from build123d import *

# Parameters (mm, degrees)
F0_R     = 1.5
F0_W     = 15
F0_H     = 49.5
F1_DEPTH = 4.5
F2_R     = 2
F3_R     = 1.5
F4_DEPTH = 2
F5_W     = 4
F5_H     = 29.5
F6_DEPTH = 6.501
F7_R     = 1.5
F8_R     = 6
F9_DEPTH = 0.5


with BuildPart() as f1:
    # F0 (on Front) → F1 (new body)
    with BuildSketch(Plane.XZ):
        with BuildLine():
            ThreePointArc((-76.25, -24.75), (-72.25, -28.75), (-68.25, -24.75))
            Line((-68.25, -24.75), (-68.25, 24.75))
            Line((-68.25, 24.75), (-68.25, 26.75))
            Line((-68.25, 26.75), (40.25, 26.75))
            Line((40.25, 26.75), (40.25, 24.75))
            Line((40.25, 24.75), (40.25, -24.75))
            ThreePointArc((40.25, -24.75), (41.4215728753, -27.5784271247), (44.25, -28.75))
            Line((44.25, -28.75), (72.25, -28.75))
            ThreePointArc((72.25, -28.75), (75.0784271247, -27.5784271247), (76.25, -24.75))
            Line((76.25, -24.75), (76.25, 27))
            ThreePointArc((76.25, 27), (75.0784271247, 29.8284271247), (72.25, 31))
            Line((72.25, 31), (-72.25, 31))
            ThreePointArc((-72.25, 31), (-75.0784271247, 29.8284271247), (-76.25, 27))
            Line((-76.25, 27), (-76.25, -24.75))
        make_face()
        with Locations((-72.25, -24.75)):
            Circle(F0_R, mode=Mode.SUBTRACT)
        with Locations((72.25, -24.75)):
            Circle(F0_R, mode=Mode.SUBTRACT)
        with Locations((60.75, 0)):
            Rectangle(F0_W, F0_H, mode=Mode.SUBTRACT)
        with Locations((-72.25, 24.75)):
            Circle(F0_R, mode=Mode.SUBTRACT)
        with Locations((72.25, 24.75)):
            Circle(F0_R, mode=Mode.SUBTRACT)
    extrude(amount=F1_DEPTH)

    # F2
    f2_edges = [f1.edges().sort_by_distance(p)[0] for p in [
        (-68.25, -2.25, -24.75),
        (40.25, -2.25, -24.75),
        (68.25, -2.25, 24.75),
        (53.25, -2.25, 24.75),
        (53.25, -2.25, -24.75),
        (68.25, -2.25, -24.75),
    ]]
    fillet(f2_edges, radius=F2_R)

    # F3 (on face) → F4 (join)
    with BuildSketch(Plane.XZ.offset(4.5)):
        with BuildLine():
            Line((-76.25, 27), (-76.25, -24.75))
            ThreePointArc((-76.25, -24.75), (-75.0784271247, -27.5784271247), (-72.25, -28.75))
            Line((-72.25, -28.75), (72.25, -28.75))
            ThreePointArc((72.25, -28.75), (75.0784271247, -27.5784271247), (76.25, -24.75))
            Line((76.25, -24.75), (76.25, 27))
            ThreePointArc((76.25, 27), (75.0784271247, 29.8284271247), (72.25, 31))
            Line((72.25, 31), (-72.25, 31))
            ThreePointArc((-72.25, 31), (-75.0784271247, 29.8284271247), (-76.25, 27))
        make_face()
        with Locations((-72.25, -24.75)):
            Circle(F3_R, mode=Mode.SUBTRACT)
        Polygon((38.25, -26.25), (-61.75, -26.25), (-61.75, 15.75), (-61.75, 26.75), (-11.75, 26.75), (-11.75, 15.75), (38.25, 15.75), align=None, mode=Mode.SUBTRACT)
        with Locations((72.25, -24.75)):
            Circle(F3_R, mode=Mode.SUBTRACT)
        with BuildLine():
            ThreePointArc((55.25, -24.75), (53.8357864376, -24.1642135624), (53.25, -22.75))
            Line((53.25, -22.75), (53.25, 22.75))
            ThreePointArc((53.25, 22.75), (53.8357864376, 24.1642135624), (55.25, 24.75))
            Line((55.25, 24.75), (66.25, 24.75))
            ThreePointArc((66.25, 24.75), (67.6642135624, 24.1642135624), (68.25, 22.75))
            Line((68.25, 22.75), (68.25, -22.75))
            ThreePointArc((68.25, -22.75), (67.6642135624, -24.1642135624), (66.25, -24.75))
            Line((66.25, -24.75), (55.25, -24.75))
        make_face(mode=Mode.SUBTRACT)
        with Locations((-72.25, 24.75)):
            Circle(F3_R, mode=Mode.SUBTRACT)
        with Locations((72.25, 24.75)):
            Circle(F3_R, mode=Mode.SUBTRACT)
    extrude(amount=F4_DEPTH)

    # F5 (on face) → F6 (cut, through all)
    with BuildSketch(Plane.XZ.offset(6.5)):
        with Locations((70.25, 0)):
            Rectangle(F5_W, F5_H)
    extrude(amount=-F6_DEPTH, mode=Mode.SUBTRACT)

    # F7
    f7_edges = [f1.edges().sort_by_distance(p)[0] for p in [
        (-11.75, -5.5, 26.75),
        (-11.75, -5.5, 15.75),
        (-61.75, -5.5, 26.75),
        (38.25, -5.5, 15.75),
        (38.25, -5.5, -26.25),
        (-61.75, -5.5, -26.25),
        (68.25, -3.25, 14.75),
        (72.25, -3.25, 14.75),
        (68.25, -3.25, -14.75),
        (72.25, -3.25, -14.75),
        (40.25, -2.25, 26.75),
        (-68.25, -2.25, 26.75),
    ]]
    fillet(f7_edges, radius=F7_R)

    # F8 (on face) → F9 (join)
    with BuildSketch(Plane.XZ.offset(6.5)):
        with Locations((-75.0784271247, 29.8284271247)):
            Circle(F8_R)
        with Locations((-75.0784271247, -27.5784271247)):
            Circle(F8_R)
        with Locations((75.0784271247, 29.8284271247)):
            Circle(F8_R)
        with Locations((75.0784271247, -27.5784271247)):
            Circle(F8_R)
    extrude(amount=-F9_DEPTH)


solid = f1.part
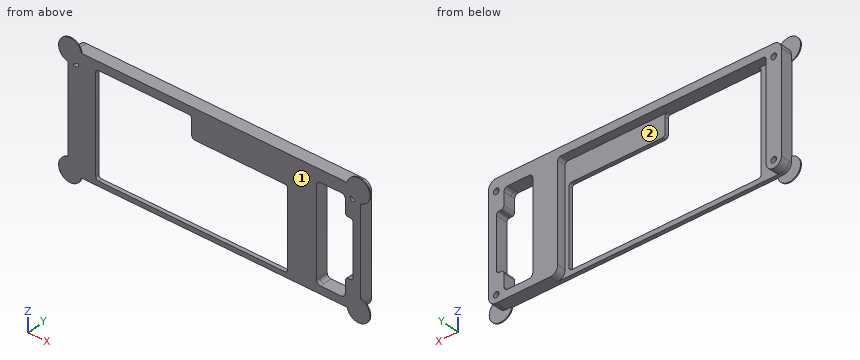
Input: part model. Units: mm. Frame: model coordinates. Face numbers are marked on the shaded views. A direction names the side the tool comes from. Coordinates: 2 decimals unless noted, no trailing zeros. Order: outer loops, then holes, each group sorted by start corner. A loop starts at its lowest first (then second) coordinate and runs counter-clockwise, first axis right, second up. Notation, with made-up numbers: M -29.75,63.5 L 14.25,63.5 A17 ccw 14.25,72.5 Z; hole C 55,15 d7. An arc over 180 degrees is marked long. Answer in a Markdown table with one row per item.
(1) Contact query for flat-ended pins moving along their axis: pin 1 Ø2 at (y, z) = (-5.5, 22.5) entering from -X; pin 2 Ø2 at (x, y) = (-27.5, -2.5) entering from -Z; pin 3 Ø2 at (x, y) = (-9, -4) entering from -Z. Output: stop coordinate, or through.
Numbers:
| item | result |
|---|---|
| pin 1 | stops at x = -76.25 |
| pin 2 | stops at z = 26.75 |
| pin 3 | stops at z = -28.75 |
(2) Section query C-C, the plane z = 21. Output: boundary loops of the cut face in (x, y), plus the area to 4 significant figures.
Numbers:
| item | result |
|---|---|
| outline | M -76.25,-6.5 L -61.75,-6.5 L -61.75,-4.5 L -68.25,-4.5 L -68.25,0 L -76.25,0 Z; M -11.75,-6.5 L 53.25,-6.5 L 53.25,0 L 40.25,0 L 40.25,-4.5 L -11.75,-4.5 Z; M 68.25,-6.5 L 76.25,-6.5 L 76.25,0 L 68.25,0 Z |
| area | 305.5 mm^2 |
(3) Material intervals for line 1 (Z direction, x = -72.25, y = -1.5); line 2 (X direction, y = -2.75, z = -16); line 3 (X direction, y = -4, z = -5), sorted ascending. Write a range as [from, to].
Numbers:
| item | result |
|---|---|
| line 1 | z = [-28.75, -26.25], [-23.25, 23.25], [26.25, 31] |
| line 2 | x = [-76.25, -68.25], [40.25, 53.25], [68.27, 76.25] |
| line 3 | x = [-76.25, -68.25], [40.25, 53.25], [72.25, 76.25] |
(4) Access query for the marked faces 1 and 2. Directions: +Z, -Z, +X, -X, +Y, -Y. A direction counts if a zero-diameter tool reaches every point of the face in a straight line with its end or side. Return the directions, or none.
Numbers:
| item | result |
|---|---|
| face 1 | +Z, -Z, +X, -X, -Y |
| face 2 | -Z, +Y |
(5) Section query D-D, the plane z = -11. Output: boundary loops of the cut face in (x, y), plus the area to 4 significant figures.
Numbers:
| item | result |
|---|---|
| outline | M -76.25,-6.5 L -61.75,-6.5 L -61.75,-4.5 L -68.25,-4.5 L -68.25,0 L -76.25,0 Z; M 38.25,-6.5 L 53.25,-6.5 L 53.25,0 L 40.25,0 L 40.25,-4.5 L 38.25,-4.5 Z; M 72.25,-6.5 L 76.25,-6.5 L 76.25,0 L 72.25,0 Z |
| area | 179.5 mm^2 |
(6) Section query B-B, the plane y = -3.5. Give the number of separate pieces and of enclosed holes in the cut face, plus the area to 3 significant figures.
Numbers:
| item | result |
|---|---|
| separate pieces | 1 |
| enclosed holes | 5 |
| area | 2,190 mm^2 |
(7) Section query A-A, the plane x = -18. Output: boundary loops of the cut face in (y, z).
Numbers:
| item | result |
|---|---|
| outline | M -6.5,-28.75 L -4.5,-28.75 L -4.5,-26.25 L -6.5,-26.25 Z; M -6.5,26.75 L 0,26.75 L 0,31 L -6.5,31 Z |
